Read the model definition and answer for the solid it produces. Units are mm, in the model's axes. A direction names the side the tool comes from. Coordinates: 2 decimals unless noted, no trailing zeros. Order: outer loops, then holes, each group sorted by start corner. A loop starts at its lowest first (then second) coordinate and runs counter-clockwise, first axis right, second up.
```python
from build123d import *

# Parameters (mm, degrees)
F2_R     = 4
F3_DEPTH = 6.5


with BuildPart() as f1:
    # F0 (on Front) → F1 (revolve)
    with BuildSketch(Plane.XZ):
        Polygon((2.75, -7), (2.75, 0), (11.15, 0), (11.15, 1), (3.65, 1), (3.65, 3), (10.55, 3), (10.55, 4), (3.05, 4), (3.05, 6.25), (10.55, 6.25), (10.55, 7.25), (3.05, 7.25), (3.05, 9.5), (10.55, 9.5), (10.55, 10.557174), (3.5, 10.557174), (3.5, 12.557174), (11, 12.557174), (11, 13.557174), (7, 13.557174), (7, 15.057174), (11, 15.057174), (11, 16.057174), (3.5, 16.057174), (3.5, 18.057174), (10.55, 18.057174), (10.55, 19.057174), (3.05, 19.057174), (3.05, 22.057174), (10.55, 22.057174), (10.55, 23.057174), (3.5, 23.057174), (3.5, 25.057174), (11, 25.057174), (11, 26.057174), (4.5, 26.057174), (4.5, 27.557174), (8, 27.557174), (8, 28.557174), (4.5, 28.557174), (4.5, 30.057174), (8, 30.057174), (8, 33.057174), (6, 33.057174), (6, 39.057174), (8, 39.057174), (8, 42.757174), (0, 42.757174), (0, 0), (0, -7), align=None)
    revolve(axis=Axis((0, 0, 21.378587), (0, 0, -1)))

    # F2 (on face) → F3 (cut)
    with BuildSketch(Plane.XY.offset(42.757174)):
        Circle(F2_R)
    extrude(amount=-F3_DEPTH, mode=Mode.SUBTRACT)


solid = f1.part
```
1) Determine the mould class of faces 4 (the cylindrical face through (-1.73, 7.81, 28.06)), 5 (the flat face through (-2.3, 2.3, 0)), 6 (the cylindrical face through (-0.59, -4.46, 26.82)), 7 (the flat face through (-7.2, -0.2, 15.057)) for opening direction Z: pulls with the +Z half, pulls with the -Z half, needs draft (parallel to the pull), parting line crosses it, or undercut.
A:
face 4: needs draft
face 5: pulls with the -Z half
face 6: undercut
face 7: undercut
2) Straight lines are drawn through the part: line 1 (Y direction, x = 0, z = 38); line 2 (Y direction, x = 0, z = 40.25); line 3 (X direction, y = -0.5, z = 37). For each, find the intervals that lie inside material, in ascending order.
A:
line 1: y = -6 to -4, 4 to 6
line 2: y = -8 to -4, 4 to 8
line 3: x = -5.98 to -3.97, 3.97 to 5.98
3) A cutting plane is placed at C-C, the plane z = 5. Determine the outline of the cut face in (x, y), and give its area (3 significant figures).
A:
outline: circle Ø6.1 at (0, 0)
area: 29.2 mm2
4) A cutting plane is placed at A-A, the plane z = 38.5. Determine the outline of the cut face in (x, y).
A:
outline: circle Ø12 at (0, 0); hole circle Ø8 at (0, 0)
5) Flat-ended cylindrical pins translate along their axes: pin 1 Ø5 at (x, z) = (-3.5, 2.5) entering from +Y; pin 2 Ø12 at (y, z) = (-6, 9.5) entering from -X; pin 3 Ø4 at (x, y) = (-4.5, 5.5) entering from -Z. Find the tip coordinate at first contact, or state that the pin passes through.
A:
pin 1: stops at y = 11.05
pin 2: stops at x = -10.97
pin 3: stops at z = 0
6) Which of the six approach directions +Z, -Z, +X, -X, +Y, -Y give full straight-line access (tool end or side, diameter ignored) to faces 1 (the flat face through (0, 0, -7)), 2 (the flat face through (0, 5, 10.557)), 3 (the cylindrical face through (-1.73, 7.81, 40.93))?
A:
face 1: -Z, +X, -X, +Y, -Y
face 2: none
face 3: +Z
7) A cutting plane is placed at B-B, the plane y = -9.5. State how many separate pieces and enclosed holes the cut face has, and give its area (3 significant figures).
A:
separate pieces: 9
enclosed holes: 0
area: 91.4 mm2
